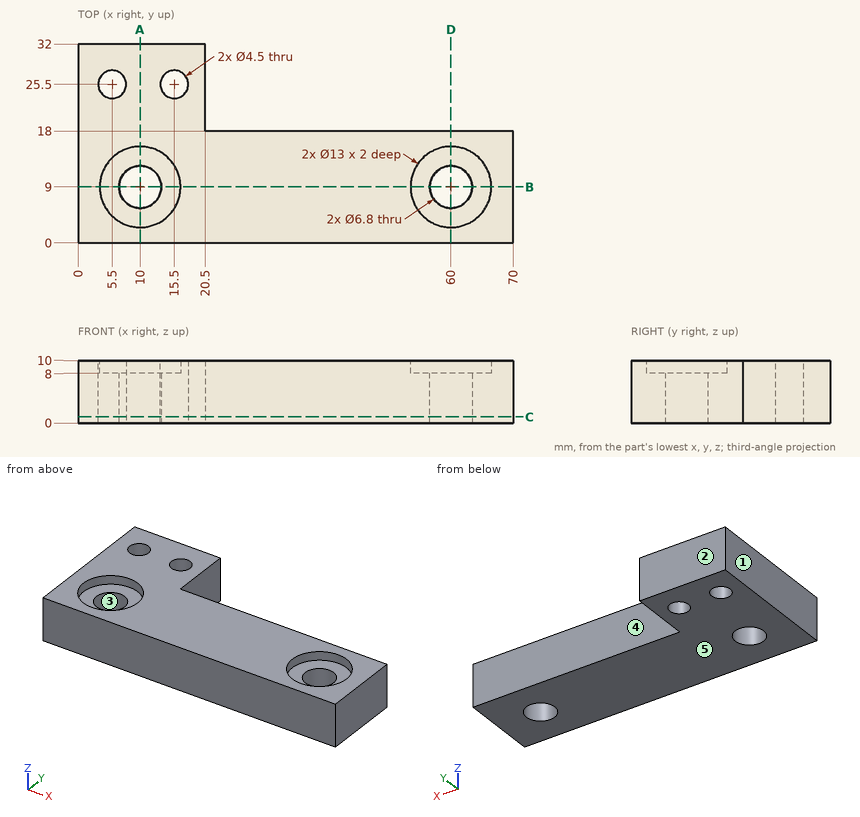
Print and shaded views of the part. All mm, measured from the part's lowest x, y and z. A direction names the side the tool comes from. Give positions to 0.01 mm unless a question says otherwise; leave off trailing zeros. Loops run counter-clockwise (first coordinate to the right, second up) from the corner with the lowest first, then second, coordinate; pieces in that order, holes last. Notation, with made-up numbers: (3.5, 82.5) -> (29.5, 82.5) arc R24 cw to (29.5, 105.5) -> close; hole circle Ø10 at (41.25, 50). An arc over 180 degrees is marked (long way). One line per question, with ' | ' between items. Start each with the question number.
1) Pin check, flat tips, straight feed: pin 1 (10.5 mm diameter, centred on x = 62, y = 10.5, fed in from +Z); pin 2 (4 mm diameter, centred on x = 5.5, y = 25.5, fed in from -Z); pin 3 (6.5 mm diameter, centred on x = 12, y = 8.5, fed in from +Z); pin 4 (2 mm diameter, centred on x = 42.5, z = 5, fed in from +Y). Stop position of each tip, or through.
2) Two-plate mould, pull along X, no slides. Class the marked faces 1, 2 and 3: released by +X, released by -X, zero draft, split by the parting line, or undercut.
3) Cut at B-B (y = 9). Give the cut face in (x, z), plus the area to 3 significant figures.
4) Cut at A-A (x = 10). Give the cut face in (y, z), plus the area to 3 significant figures.
5) 3-axis set-ups, long thin cutter, end or side, ignore diameter. For the marked faces 4 and 5: which of +Z, -Z, +X, -X, +Y, -Y reach the whole face in a straight line?
6) Cut at C-C (z = 1). Give the cut face in (x, y), plus the area to 3 significant figures.
7) Probe L1, parallel to X at y = 9, z = 4; L2, parallel to Y at x = 5.5, z = 4; L3, parallel to X at y = 10, z = 8.5. List the from-to ranges inside material, lowest first.
8) Cut at D-D (x = 60). Give the cut face in (y, z), plus the area to 3 significant figures.
Return value:
1) pin 1: z = 10 | pin 2: through | pin 3: z = 8 | pin 4: y = 18
2) face 1: released by -X | face 2: zero draft | face 3: undercut
3) outline: (0, 0) -> (6.6, 0) -> (6.6, 8) -> (3.5, 8) -> (3.5, 10) -> (0, 10) -> close; (13.4, 0) -> (56.6, 0) -> (56.6, 8) -> (53.5, 8) -> (53.5, 10) -> (16.5, 10) -> (16.5, 8) -> (13.4, 8) -> close; (63.4, 0) -> (70, 0) -> (70, 10) -> (66.5, 10) -> (66.5, 8) -> (63.4, 8) -> close | area: 539 mm^2
4) outline: (0, 0) -> (5.6, 0) -> (5.6, 8) -> (2.5, 8) -> (2.5, 10) -> (0, 10) -> close; (12.4, 0) -> (32, 0) -> (32, 10) -> (15.5, 10) -> (15.5, 8) -> (12.4, 8) -> close | area: 240 mm^2
5) face 4: +Z, -Z, +X, +Y | face 5: -Z, +X, -X, +Y, -Y
6) outline: (0, 0) -> (70, 0) -> (70, 18) -> (20.5, 18) -> (20.5, 32) -> (0, 32) -> close; hole circle Ø4.5 at (5.5, 25.5); hole circle Ø6.8 at (10, 9); hole circle Ø4.5 at (15.5, 25.5); hole circle Ø6.8 at (60, 9) | area: 1,440 mm^2
7) L1: 0 to 6.6, 13.4 to 56.6, 63.4 to 70 | L2: 0 to 23.25, 27.75 to 32 | L3: 0 to 3.58, 16.42 to 53.58, 66.42 to 70
8) outline: (0, 0) -> (5.6, 0) -> (5.6, 8) -> (2.5, 8) -> (2.5, 10) -> (0, 10) -> close; (12.4, 0) -> (18, 0) -> (18, 10) -> (15.5, 10) -> (15.5, 8) -> (12.4, 8) -> close | area: 99.6 mm^2
